```python
from build123d import *

# Parameters (mm, degrees)
F0_R     = 30.1625
F1_DEPTH = 3.175
F3_DEPTH = 6.35
F4_R     = 2.75
F5_DEPTH = 25.4


with BuildPart() as f1:
    # F0 (on Top) → F1 (new body)
    with BuildSketch(Plane.XY):
        Circle(F0_R)
    extrude(amount=F1_DEPTH)

    # F2 (on face) → F3 (join)
    with BuildSketch(Plane.XY.offset(3.175)):
        with BuildLine():
            ThreePointArc((-12.747223, -23.787254), (-26.9875, 0), (-12.747223, 23.787254))
            Line((-12.747223, 23.787254), (-12.747223, 27.336509))
            ThreePointArc((-12.747223, 27.336509), (-30.1625, 0), (-12.747223, -27.336509))
            Line((-12.747223, -27.336509), (-12.747223, -23.787254))
        make_face()
        with BuildLine():
            ThreePointArc((30.1625, 0), (25.438794, 16.206299), (12.747223, 27.336509))
            Line((12.747223, 27.336509), (12.747223, 23.787254))
            ThreePointArc((12.747223, 23.787254), (26.9875, 0), (12.747223, -23.787254))
            Line((12.747223, -23.787254), (12.747223, -27.336509))
            ThreePointArc((12.747223, -27.336509), (25.438794, -16.206299), (30.1625, 0))
        make_face()
    extrude(amount=F3_DEPTH)

    # F4 (on face) → F5 (cut)
    with BuildSketch(Plane(origin=(0, 0, 0), x_dir=(1, 0, 0), z_dir=(0, 0, -1))):
        with BuildLine():
            Line((6.858, 17.6022), (-6.858, 17.6022))
            ThreePointArc((-6.858, 17.6022), (-8.636, 15.8242), (-6.858, 14.0462))
            Line((-6.858, 14.0462), (6.858, 14.0462))
            ThreePointArc((6.858, 14.0462), (8.636, 15.8242), (6.858, 17.6022))
        make_face()
        with BuildLine():
            ThreePointArc((6.858, -17.6022), (8.636, -15.8242), (6.858, -14.0462))
            Line((6.858, -14.0462), (-6.858, -14.0462))
            ThreePointArc((-6.858, -14.0462), (-8.636, -15.8242), (-6.858, -17.6022))
            Line((-6.858, -17.6022), (6.858, -17.6022))
        make_face()
        Circle(F4_R)
        with BuildLine():
            ThreePointArc((-6.858, 4.7625), (-5.735468, 5.227468), (-5.2705, 6.35))
            ThreePointArc((-5.2705, 6.35), (-5.735468, 7.472532), (-6.858, 7.9375))
            ThreePointArc((-6.858, 7.9375), (-8.4455, 6.35), (-6.858, 4.7625))
        make_face()
        with BuildLine():
            ThreePointArc((-6.858, 7.9375), (-5.735468, 7.472532), (-5.2705, 6.35))
            ThreePointArc((-5.2705, 6.35), (-5.735468, 5.227468), (-6.858, 4.7625))
            Line((-6.858, 4.7625), (6.858, 4.7625))
            ThreePointArc((6.858, 4.7625), (5.2705, 6.35), (6.858, 7.9375))
            Line((6.858, 7.9375), (-6.858, 7.9375))
        make_face()
        with BuildLine():
            ThreePointArc((8.4455, 6.35), (7.980532, 7.472532), (6.858, 7.9375))
            ThreePointArc((6.858, 7.9375), (5.2705, 6.35), (6.858, 4.7625))
            ThreePointArc((6.858, 4.7625), (7.980532, 5.227468), (8.4455, 6.35))
        make_face()
        with BuildLine():
            Line((6.858, -4.7625), (-6.858, -4.7625))
            ThreePointArc((-6.858, -4.7625), (-5.735468, -5.227468), (-5.2705, -6.35))
            ThreePointArc((-5.2705, -6.35), (-5.735468, -7.472532), (-6.858, -7.9375))
            Line((-6.858, -7.9375), (6.858, -7.9375))
            ThreePointArc((6.858, -7.9375), (5.2705, -6.35), (6.858, -4.7625))
        make_face()
        with BuildLine():
            ThreePointArc((-5.2705, -6.35), (-5.735468, -5.227468), (-6.858, -4.7625))
            ThreePointArc((-6.858, -4.7625), (-8.4455, -6.35), (-6.858, -7.9375))
            ThreePointArc((-6.858, -7.9375), (-5.735468, -7.472532), (-5.2705, -6.35))
        make_face()
        with BuildLine():
            ThreePointArc((8.4455, -6.35), (7.980532, -5.227468), (6.858, -4.7625))
            ThreePointArc((6.858, -4.7625), (5.2705, -6.35), (6.858, -7.9375))
            ThreePointArc((6.858, -7.9375), (7.980532, -7.472532), (8.4455, -6.35))
        make_face()
    extrude(amount=-F5_DEPTH, mode=Mode.SUBTRACT)


solid = f1.part
```
Input: part model. Units: mm. Frame: model coordinates. A direction names the side the tool comes from. Round coordinates to 2 decimals unless told otherwise and drop trailing zeros. Loops run counter-clockwise (first coordinate to the right, second up) from the corner with the lowest first, then second, coordinate; pieces in that order, holes last. Notation, with made-up numbers: (9.5, 0.25) -> (40.5, 0.25) arc R11 cw to (40.5, 20.25) -> close; hole circle Ø11 at (-24.5, 10). An arc over 180 degrees is marked (long way). One line per item, written item: value.
(1) Section D-D (y = 16). Return the cut outline in (x, z) (3 decimals).
Geometry check:
outline: (-25.569, 0) -> (-8.627, 0) -> (-8.627, 3.175) -> (-21.733, 3.175) -> (-21.733, 9.525) -> (-25.569, 9.525) -> close; (8.627, 0) -> (25.569, 0) -> (25.569, 9.525) -> (21.733, 9.525) -> (21.733, 3.175) -> (8.627, 3.175) -> close
(2) Section B-B (z = 8.5). Return the cut outline in (x, y) (1 decimal).
Geometry check:
outline: (-12.7, -27.3) -> (-12.7, -23.8) arc R27 cw to (-12.7, 23.8) -> (-12.7, 27.3) arc R30.2 ccw to start; (12.7, -27.3) arc R30.2 ccw to (30.2, 0) arc R30.2 ccw to (12.7, 27.3) -> (12.7, 23.8) arc R27 cw to (12.7, -23.8) -> close
(3) Pin query (flat end, axial travel): pin 1 (16 mm diameter, centred on x = -9, y = -14, fed in from +Z) (3 decimals); pin 2 (1 mm diameter, centred on y = 2, z = 3.5, fed in from +X); pin 3 (1.8 mm diameter, centred on y = 26, z = 7.5, fed in from -X). Return the tip coordinate at first contact, or that it passes through.
Geometry check:
pin 1: z = 3.175
pin 2: x = 30.13
pin 3: x = -16.73
(4) Set-up query: faces 1 (the face through (26.984, 0.408, 6.306)), 2 (the face through (-27.3, 0.1, 9.525)), 3 (the face through (0, 7.938, 2)), 4 (the face through (12.747, -26, 6)). Return all of +Z, -Z, +X, -X, +Y, -Y with unobstructed straight access to the full face (end or side cutting, diameter ignored); none if empty.
Geometry check:
face 1: +Z
face 2: +Z, +X, -X, +Y, -Y
face 3: +Z, -Z
face 4: +Z, +Y, -Y
(5) Section A-A (x = 0). Give the number of separate pieces and of enclosed holes in the cut face, plus the area to 3 significant figures.
Geometry check:
separate pieces: 6
enclosed holes: 0
area: 131 mm2
(6) Mould query, pull axis Y, two halves, no side actions, for faces 5 (the face through (0, -4.762, 2)), 6 (the face through (6, 0, 3.175)), 7 (the face through (-12.747, 26, 6)). Classes: pulls with the +Y half, pulls with the -Y half, needs draft (parallel to the pull), parting line crosses it, or undercut.
Geometry check:
face 5: undercut
face 6: undercut
face 7: needs draft
(7) Material intervals for line 1 (Y direction, x = 0, z = 1.6); line 2 (X direction, y = 0, z = 1.65); line 3 (Z direction, x = 20, y = -6) (3 decimals), sorted ascending. Write a range as [from, to].
Geometry check:
line 1: [-30.16, -17.6], [-14.05, -7.94], [-4.76, -2.75], [2.75, 4.76], [7.94, 14.05], [17.6, 30.16]
line 2: [-30.16, -2.75], [2.75, 30.16]
line 3: [0, 3.175]
